Input: part model. Units: mm. Frame: model coordinates. A direction names the side the tool comes from. Give positions to 0.01 mm unless a question says otherwise; leave off trailing zeros. Write each loop counter-clockwise with the first axis right and the second up, starting at its lowest first coordinate (ties: lowest second). Pieces come first, ordered by that corner, then holes. Notation, with made-up numbers: (-36, -4) - (-10, -4) arc R10 ccw to (-10, 3) - close; hole circle Ø11 at (8.25, 89.25). An arc over 180 degrees is marked (long way). Use a Markdown table: item, result. Add a question column.
1. Pin query (flat end, axial travel): pin 1 (5 mm diameter, centred on x = -56, z = -8.5, fed in from -Y). Return the tip coordinate at first contact, or that it passes through.
2. Set-up query: faces 1 (the cylindrical face through (232.947, -102.451, -5.916)), 2 (the flat face through (-295.5, -193, -6)). Return all of +Z, -Z, +X, -X, +Y, -Y with unobstructed straight access to the full face (end or side cutting, diameter ignored); none if empty.
3. Section query B-B, the plane z = -9.75. Return loops of the section in (x, y).
4. Section query A-A, the plane y = -39.5. Return loops of the section in (x, z), plus the area to 3 significant figures.
5. Material intervals for probe 1 along Y at (x, z) = (-241, -5.5); probe 2 along Y at (x, z) = (209, -1.25); probe 3 along Y at (x, z) = (-41, -1.75), sorted ascending.
6. Mould query, pull axis X, two halves, no side actions, for faces 3 (the cylindrical face through (-281.818, -12.975, -5.916)), 4 (the flat face through (178.592, -121.915, -5.916)), 5 (the flat face through (-3, 0, -6)). Classes: released by +X, released by -X, zero draft, split by the parting line, or undercut.
7. Section query C-C, the plane x = -106. Return loops of the section in (y, z), plus the area to 3 significant figures.
```python
from build123d import *

# Parameters (mm, degrees)
PAD_DEPTH       = 12
POCKET_DEPTH    = 12
POCKET001_DEPTH = 12


with BuildPart() as part:
    # Sketch → Pad (new body)
    with BuildSketch(Plane.XY):
        with BuildLine():
            Line((-250, 0), (250, 0))
            ThreePointArc((295.5, -45.5), (282.173358544, -13.326641456), (250, 0))
            Line((295.5, -45.5), (295.5, -335.5))
            ThreePointArc((225, -387.5984644687), (273.3901991349, -379.3306399679), (295.5, -335.5))
            ThreePointArc((225, -387.5984644687), (0, -351), (-225, -387.5984644687))
            ThreePointArc((-295.5, -335.5), (-273.3901991349, -379.3306399679), (-225, -387.5984644687))
            Line((-295.5, -335.5), (-295.5, -45.5))
            ThreePointArc((-250, 0), (-282.173358544, -13.326641456), (-295.5, -45.5))
        make_face()
    extrude(amount=-PAD_DEPTH)

    # Sketch001 → Pocket (cut)
    with BuildSketch(Plane.XY):
        with BuildLine():
            ThreePointArc((-136.5, -30), (-146, -39.5), (-136.5, -49))
            Line((-136.5, -49), (-20, -49))
            ThreePointArc((-20, -49), (0, -69), (20, -49))
            Line((155.5000159433, -49), (20, -49))
            ThreePointArc((155.5000159433, -49), (165, -39.4999920284), (155.5, -30))
            Line((155.5, -30), (-136.5, -30))
        make_face()
    extrude(amount=-POCKET_DEPTH, mode=Mode.SUBTRACT)

    # Sketch002 → Pocket001 (cut)
    with BuildSketch(Plane.XY):
        with BuildLine():
            ThreePointArc((256.3808583259, -139.7068088046), (232.3192402672, -102.2162961861), (189.7885344689, -115.4691850901))
            Line((189.7885344689, -115.4691850901), (181.973144238, -112.6246156768))
            Line((175.3037514432, -130.9486217822), (181.973144238, -112.6246156768))
            Line((175.3037514432, -130.9486217822), (183.1191416741, -133.7931911954))
            ThreePointArc((183.1191416741, -133.7931911954), (207.1807597328, -171.2837038139), (249.7114655311, -158.0308149099))
            Line((257.526855762, -160.8753843232), (249.7114655311, -158.0308149099))
            Line((264.1962485568, -142.5513782178), (257.526855762, -160.8753843232))
            Line((256.3808583259, -139.7068088046), (264.1962485568, -142.5513782178))
        make_face()
    extrude(amount=-POCKET001_DEPTH, mode=Mode.SUBTRACT)


solid = part.part
```
Result sheet:
| question | item | result |
|---|---|---|
| 1 | pin 1 | stops at y = -353.41 |
| 2 | face 1 | +Z, -Z |
| 2 | face 2 | +Z, -Z, -X, +Y, -Y |
| 3 | outline | (-295.5, -335.5) arc R54.5 ccw to (-225, -387.6) arc R709.93 cw to (225, -387.6) arc R54.5 ccw to (295.5, -335.5) - (295.5, -45.5) arc R45.5 ccw to (250, 0) - (-250, 0) arc R45.5 ccw to (-295.5, -45.5) - close; hole (-136.5, -49) - (-20, -49) arc R20 ccw to (20, -49) - (155.5, -49) arc R9.5 ccw to (155.5, -30) - (-136.5, -30) arc R9.5 ccw to start; hole (175.3, -130.95) - (183.12, -133.79) arc R36.75 ccw to (249.71, -158.03) - (257.53, -160.88) - (264.2, -142.55) - (256.38, -139.71) arc R36.75 ccw to (189.79, -115.47) - (181.97, -112.62) - close |
| 4 | outline | (-295.1, -12) - (-146, -12) - (-146, 0) - (-295.1, 0) - close; (165, -12) - (295.1, -12) - (295.1, 0) - (165, 0) - close |
| 4 | area | 3,350 mm² |
| 5 | probe 1 | y = -390 to 0 |
| 5 | probe 2 | y = -382.46 to -171.89, -101.61 to 0 |
| 5 | probe 3 | y = -352.18 to -49, -30 to 0 |
| 6 | face 3 | released by -X |
| 6 | face 4 | undercut |
| 6 | face 5 | zero draft |
| 7 | outline | (-358.96, -12) - (-49, -12) - (-49, 0) - (-358.96, 0) - close; (-30, -12) - (0, -12) - (0, 0) - (-30, 0) - close |
| 7 | area | 4,080 mm² |
